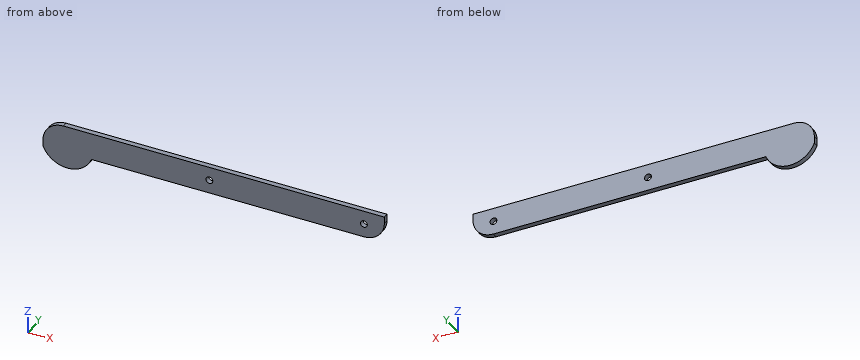
```python
from build123d import *

# Parameters (mm, degrees)
SKETCH1_R           = 12.7
BOSS_EXTRUDE1_DEPTH = 19.05


with BuildPart() as part:
    # Sketch1 → Boss-Extrude1 (new body)
    with BuildSketch(Plane(origin=(0, 0, 0), x_dir=(1, 0, 0), z_dir=(0, 1, 0))):
        with BuildLine():
            Line((-558.8, -50.8), (635, -50.8))
            Line((635, -50.8), (635, -25.4))
            ThreePointArc((635, -25.4), (612.681536726, 28.481536726), (558.8, 50.8))
            Line((558.8, 50.8), (-454.65655736, 50.8))
            ThreePointArc((-454.65655736, 50.8), (-544.82827868, 112.124515873), (-635, 50.8))
            Line((-635, 50.8), (-635, 25.4))
            ThreePointArc((-635, 25.4), (-612.681536726, -28.481536726), (-558.8, -50.8))
        make_face()
        with Locations((-15.94, 0)):
            Circle(SKETCH1_R, mode=Mode.SUBTRACT)
        with Locations((558.8, 0)):
            Circle(SKETCH1_R, mode=Mode.SUBTRACT)
    extrude(amount=BOSS_EXTRUDE1_DEPTH)


solid = part.part
```
Can you work these out from the model? Positions are in its coordinate system, mm. Give positions to 0.01 mm unless a question says otherwise; leave off trailing zeros. Write each loop counter-clockwise with the first axis right and the second up, starting at its lowest first coordinate (ties: lowest second). Pieces come first, ordered by that corner, then holes. Notation, with made-up numbers: (77.25, 61) - (126.25, 61) arc R17 ccw to (126.25, 90) - close; hole circle Ø9 at (20, -39.75). An arc over 180 degrees is marked (long way). Write item = value, one per line. Start each with the question number.
1. Imagine slicing it at D-D (z = -71). Please give me the cut outline in (x, y).
2. Imagine slicing it at A-A (y = 11.25). Please give me the cut outline in (x, z).
3. For pin 1 (2 mm diameter, centred on y = 9.5, z = -4, fed in from -X); pin 2 (3 mm diameter, centred on x = -452.5, z = -26, fed in from -Y); pin 3 (1.5 mm diameter, centred on x = 351.5, y = 8.5, fed in from -Z); pin 4 (3 mm diameter, centred on y = 7.5, z = -62.5, fed in from -X), each with a flat end and sliding along its axis, tell me the tip position at first contact or that it passes through.
4. Please list where these lines run through material, in increasing order: line 1 (Z direction, x = -15.94, y = 9.5); line 2 (X direction, y = 14, z = 0); line 3 (X direction, y = 7, z = 6.5).
5. Imagine slicing it at B-B (x = -15.94). Please give me the cut outline in (y, z).
6. Imagine slicing it at C-C (z = 0). Please give me the cut outline in (x, y).
Worked answers:
q1.outline = (-624.1, 0) - (-465.56, 0) - (-465.56, 19.05) - (-624.1, 19.05) - close
q2.outline = (-635, -50.8) arc R96.96 ccw to (-454.66, -50.8) - (558.8, -50.8) arc R76.2 ccw to (635, 25.4) - (635, 50.8) - (-558.8, 50.8) arc R76.2 ccw to (-635, -25.4) - close; hole circle Ø25.4 at (-15.94, 0); hole circle Ø25.4 at (558.8, 0)
q3.pin_1 = -632.22
q3.pin_2 = 0
q3.pin_3 = -50.8
q3.pin_4 = -630.27
q4.line_1 = -50.8 to -12.7, 12.7 to 50.8
q4.line_2 = -630.64 to -28.64, -3.24 to 546.1, 571.5 to 630.64
q4.line_3 = -628 to -26.85, -5.03 to 547.89, 569.71 to 632.62
q5.outline = (0, -50.8) - (19.05, -50.8) - (19.05, -12.7) - (0, -12.7) - close; (0, 12.7) - (19.05, 12.7) - (19.05, 50.8) - (0, 50.8) - close
q6.outline = (-630.64, 0) - (-28.64, 0) - (-28.64, 19.05) - (-630.64, 19.05) - close; (-3.24, 0) - (546.1, 0) - (546.1, 19.05) - (-3.24, 19.05) - close; (571.5, 0) - (630.64, 0) - (630.64, 19.05) - (571.5, 19.05) - close
